Read the model definition and answer for the solid it produces. Units are mm, in the model's axes. A direction names the side the tool comes from. Coordinates: 2 decimals unless noted, no trailing zeros. Write each loop counter-clockwise with the first axis right and the second up, starting at its lowest first coordinate (ties: lowest second). Pieces come first, ordered by that corner, then holes. Notation, with made-up numbers: (85.25, -10.5) -> (110.25, -10.5) arc R13 cw to (110.25, 0.5) -> close; hole circle Ø2 at (34.25, 52). An arc over 180 degrees is marked (long way). Use CSV: the item, a comma, the result in double quotes.
from build123d import *

# Parameters (mm, degrees)
SKETCH_R     = 2.8
PAD_DEPTH    = 3
SKETCH001_R  = 1.45
PAD001_DEPTH = 10
POCKET_DEPTH = 2
CHAMFER_SIZE = 0.25


with BuildPart() as part:
    # Sketch → Pad (new body)
    with BuildSketch(Plane.XY):
        Circle(SKETCH_R)
    extrude(amount=PAD_DEPTH)

    # Sketch001 (on Face3 of Pad) → Pad001 (join)
    with BuildSketch(Plane.XY.offset(3)):
        Circle(SKETCH001_R)
    extrude(amount=PAD001_DEPTH)

    # Sketch002 (on Face2 of Pad001) → Pocket (cut)
    with BuildSketch(Plane(origin=(0, 0, 0), x_dir=(1, 0, 0), z_dir=(0, 0, -1))):
        Polygon((1.259542, 0.814588), (-0.075682, 1.49809), (-1.335225, 0.683502), (-1.259542, -0.814588), (0.075682, -1.49809), (1.335225, -0.683502), align=None)
    extrude(amount=-POCKET_DEPTH, mode=Mode.SUBTRACT)

    # Chamfer
    chamfer_edges = [part.edges().sort_by_distance(p)[0] for p in [
        (-2.8, 0, 3),
        (-2.8, 0, 0),
        (1.297384, -0.065543, 0),
        (0.705454, 1.090796, 0),
        (-0.59193, 1.156339, 0),
        (-1.297384, 0.065543, 0),
        (-0.705454, -1.090796, 0),
        (0.59193, -1.156339, 0),
        (-1.45, 0, 13),
    ]]
    chamfer(chamfer_edges, length=CHAMFER_SIZE)


solid = part.part
1. Find the intervals of material crossed by line 1 along Z through (x, y) = (1.25, 0.95); line 2 along Y through (x, z) = (0.1, 7.25); line 3 along X through (y, z) = (-1.2, 12.25), in increasing order.
Solutions:
line 1,"z = 0.07 to 3"
line 2,"y = -1.45 to 1.45"
line 3,"x = -0.81 to 0.81"
2. For a pull along Y with two mould halves and no side action, classify faces 1 (the flat face through (-0.6, 1.15, 1.11)), 2 (the flat face through (2, 0, 0)), 3 (the cylindrical face through (-1.45, 0.06, 7.81)), 4 (the flat face through (-0.659, 1.26, 0.127)) as pulls with the +Y half, pulls with the -Y half, needs draft (parallel to the pull), parting line crosses it, or undercut.
Solutions:
face 1,"undercut"
face 2,"needs draft"
face 3,"parting line crosses it"
face 4,"undercut"
3. A tool of negligible diameter and unlimited length cuts with its end or side. For faces 5 (the flat face through (-1.298, 0.055, 1.113)), 6 (the flat face through (0, -2, 3)), 7 (the cylindrical face through (-2.8, 0.1, 1.5)), from which of +Z, -Z, +X, -X, +Y, -Y can it reach the whole face along a straight path? Write none if from no direction.
Solutions:
face 5,"-Z"
face 6,"+Z"
face 7,"+Z, -Z"
4. Each of these flat-tipped pins is pushed along its axis until it touches: pin 1 Ø1.5 at (y, z) = (1, 1.5) entering from +X; pin 2 Ø1.5 at (x, z) = (-1, 4) entering from -Y; pin 3 Ø3 at (x, y) = (-2, 2) entering from +Z. Where does it stop, or does it pass through?
Solutions:
pin 1,"stops at x = 2.79"
pin 2,"stops at y = -1.43"
pin 3,"stops at z = 12.87"
5. A cutting plane is placed at A-A (z = 6). Give the vertices of the cut face in (x, y), and give its area (3 significant figures).
Solutions:
outline,"circle Ø2.9 at (0, 0)"
area,"6.61 mm^2"
